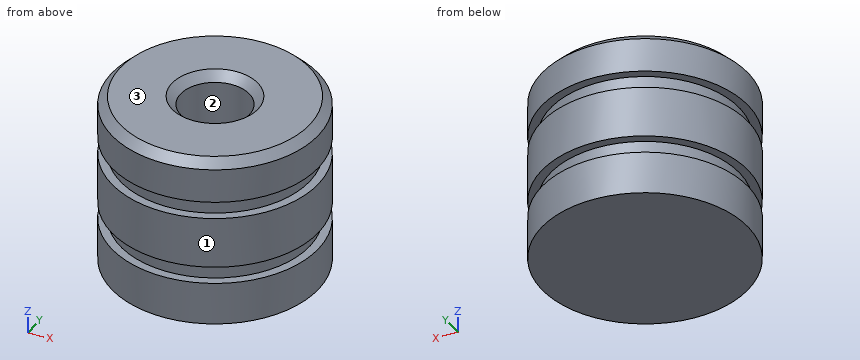
Solid Edge part; units mm, degrees
sketch "Sketch1" plane through (0, 0, 0) normal (0, 0, 1) x (1, 0, 0)
  circle A0 centre (0, 0) radius 6
extrude "Protrusion1" add sketch "Sketch1" along normal mid plane 10
sketch "Sketch2" plane through (0, 0, 0) normal (1, 0, 0) x (0, 1, 0)
  line L0 (5.5, 1.5) -> (6, 1.5)
  line L1 (6, 2.5) -> (6, 1.5)
  line L2 (6, 2.5) -> (5.5, 2.5)
revolve "RevolvedCutout1" cut sketch "Sketch2" angle 360 about axis through (0, 0, 6.6251) along (0, 0, -1) material side at (0, 5.75, 1.55)
sketch "Sketch3" plane through (0, 0, 2.5) normal (0, 0, -1) x (1, 0, 0)
  circle A0 centre (0, 0) radius 5.5
extrude "ExtrudedProtrusion_2" add sketch "Sketch3" along normal blind 1
sketch "Sketch4" plane through (0, 0, 0) normal (1, 0, 0) x (0, 1, 0)
  line L0 (6, -2.5) -> (5.5, -2.5)
  line L1 (6, -1.5) -> (6, -2.5)
  line L2 (5.5, -1.5) -> (6, -1.5)
revolve "RevolvedCutout2" cut sketch "Sketch4" angle 360 about axis through (0, 0, 6.6251) along (0, 0, -1) material side at (0, 5.75, -2.45)
mirror "Mirror1" about plane through (0, 0, 0) normal (0, 0, 1) of "ExtrudedProtrusion_2"
chamfer "Chamfer_1" distance 0.5 angle 45 1 edges at (-6, 0, 5)
hole "Hole_1" at (0, 0, 5) direction (0, 0, -1) diameter 4 depth 8 countersink diameter 5 countersink angle 90
cosmetic_thread "Thread_1" thread depth 7.5
Verification items for the finished model (mm, model axes). Face numbers are marked on the shaded views. Give positions to 0.01 mm unless a question says otherwise; leave off trailing zeros. Order: outer loops, then holes, each group sorted by start corner. A loop starts at its lowest first (then second) coordinate and runs counter-clockwise, first axis right, second up. Notation, with made-up numbers: (30, 40.25) -> (48, 40.25) arc R16 ccw to (48, 61.25) -> close; hole circle Ø3 at (36, 33.5). An arc over 180 degrees is marked (long way). Use a Markdown table: item, result.
1) Mould release check, pull along Y, two halves, no side actions. Record for the marked faces 1, 2 and 3: pulls with the +Y half, pulls with the -Y half, needs draft (parallel to the pull), parting line crosses it, or undercut.
Results:
| item | result |
|---|---|
| face 1 | parting line crosses it |
| face 2 | undercut |
| face 3 | needs draft |
2) Section check D-D, the plane z = -3.25. Record the boundary of the cut face in (x, y), then the cut area to 3 significant figures.
Results:
| item | result |
|---|---|
| outline | circle Ø12 at (0, 0) |
| area | 113 mm² |
3) Material ranges on probe 1 along Y at (x, z) = (0, -0.25); probe 2 along X at (y, z) = (0, 1.75), recorded low to high.
Results:
| item | result |
|---|---|
| probe 1 | -6 to -2, 2 to 6 |
| probe 2 | -5.5 to -2, 2 to 5.5 |
4) Depth check by flat-ended pin: pin 1 Ø3.5 at (x, y) = (0, 0) entering from +Z; pin 2 Ø2 at (y, z) = (-2, 3.5) entering from -X; pin 3 Ø2 at (y, z) = (-4, 1) entering from -X. Enter the tip coordinate at first touch or a pass-through.
Results:
| item | result |
|---|---|
| pin 1 | z = -3 |
| pin 2 | x = -5.92 |
| pin 3 | x = -5.2 |
5) Section check A-A, the plane x = 0. Record the boundary of the cut face in (y, z).
Results:
| item | result |
|---|---|
| outline | (-6, -5) -> (6, -5) -> (6, -2.5) -> (5.5, -2.5) -> (5.5, -1.5) -> (6, -1.5) -> (6, 1.5) -> (5.5, 1.5) -> (5.5, 2.5) -> (6, 2.5) -> (6, 4.5) -> (5.5, 5) -> (2.5, 5) -> (2, 4.5) -> (2, -3) -> (-2, -3) -> (-2, 4.5) -> (-2.5, 5) -> (-5.5, 5) -> (-6, 4.5) -> (-6, 2.5) -> (-5.5, 2.5) -> (-5.5, 1.5) -> (-6, 1.5) -> (-6, -1.5) -> (-5.5, -1.5) -> (-5.5, -2.5) -> (-6, -2.5) -> close |
6) Section check C-C, the plane z = -0.75. Record the boundary of the cut face in (x, y).
Results:
| item | result |
|---|---|
| outline | circle Ø12 at (0, 0); hole circle Ø4 at (0, 0) |
